Autodesk Inventor part; units mm, degrees
ref_plane "YZ Plane" through (0, 0, 0) normal (1, 0, 0) x (0, 1, 0)
ref_plane "XZ Plane" through (0, 0, 0) normal (0, 1, 0) x (-1, 0, 0)
ref_plane "XY Plane" through (0, 0, 0) normal (0, 0, 1) x (1, 0, 0)
sketch "Szkic1" plane through (0, 0, 0) normal (0, 0, 1) x (1, 0, 0)
  line L0 (11.5, -11.5) -> (-11.5, -11.5)
  line L1 (-11.5, -11.5) -> (-11.5, 11.5)
  line L2 (-11.5, 11.5) -> (11.5, 11.5)
  line L3 (11.5, 11.5) -> (11.5, -11.5)
  line L4 (11.5, -11.5) -> (-11.5, 11.5) construction
  line L5 (-11.5, -11.5) -> (11.5, 11.5) construction
  point P0 (0, 0)
  dimension "d0" = 23
  dimension "d1" = 23
extrude "Wyciągnięcie proste1" add sketch "Szkic1" along normal blind 23
fillet "Zaokrąglenie1" radius 0.5 12 edges at (0, 11.5, 23) (11.5, 11.5, 11.5) (11.5, 0, 23) (11.5, 0, 0) (11.5, -11.5, 11.5) (0, -11.5, 23) (0, -11.5, 0) (-11.5, -11.5, 11.5) (0, 11.5, 0) (-11.5, 11.5, 11.5) (-11.5, 0, 0) (-11.5, 0, 23)
sketch "Szkic2" plane through (0, 0, 23) normal (0, 0, 1) x (1, 0, 0)
  circle A0 centre (0, 0) radius 1.75
  circle A1 centre (0, 0) radius 2.25
  dimension "d5" = 3.5
  dimension "d6" = 4.5
extrude "Wyciągnięcie proste2" add sketch "Szkic2" along normal blind 1
fillet "Zaokrąglenie2" radius 1 1 edges at (-2.25, 0, 23)
properties part number "Kamera"
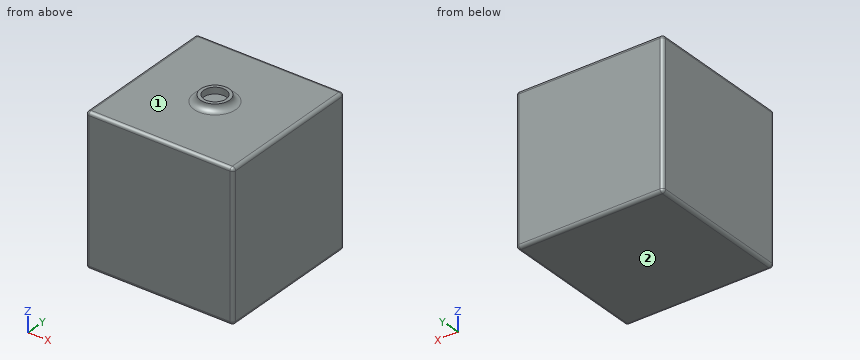
Work out the finished part from the listing and answer in its coordinate system (mm). Face numbers are marked on the shaded views. A direction names the side the tool comes from. Give positions to 0.01 mm unless a question says otherwise; leave off trailing zeros. Order: outer loops, then holes, each group sorted by start corner. A loop starts at its lowest first (then second) coordinate and runs counter-clockwise, first axis right, second up. Notation, with made-up numbers: M 1.25,49.25 L 24.25,49.25 A6 ccw 24.25,58.25 Z; hole C -9,-29.5 d2. An arc over 180 degrees is marked long. Return JSON: item names as keys, results as strings.
1) A tool of negligible diameter and unlimited length cuts with its end or side. For the marked faces 1 and 2, from which of +Z, -Z, +X, -X, +Y, -Y can it reach the whole face along a straight path? Write none if from no direction.
Resolved:
{"face 1": "+Z", "face 2": "-Z, +X, -X, +Y, -Y"}
2) Section A-A, the plane x = 4.75 is taken. Write down the section's boundary in (y, z), plus the area to 3 significant figures.
Resolved:
{"outline": "M -11.5,0.5 A0.5 ccw -11,0 L 11,0 A0.5 ccw 11.5,0.5 L 11.5,22.5 A0.5 ccw 11,23 L -11,23 A0.5 ccw -11.5,22.5 Z", "area": "529 mm^2"}
3) Straight lines are drawn through the part: line 1 along Z through (x, y) = (1.25, 1); line 2 along Y through (x, z) = (0, 23.7); line 3 along Y through (x, z) = (0, 23.3). For each, find the intervals that lie inside material, in ascending order. Write a range as [from, to].
Resolved:
{"line 1": "[0, 23]", "line 2": "[-2.3, -1.75], [1.75, 2.3]", "line 3": "[-2.54, -1.75], [1.75, 2.54]"}
4) Each of these flat-tipped pins is pushed along its axis until it touches: pin 1 (5 mm diameter, centred on x = 6.5, y = 1.5, fed in from -Z); pin 2 (1 mm diameter, centred on x = 0, y = 0.5, fed in from +Z); pin 3 (6.5 mm diameter, centred on x = -4, y = 4.5, fed in from +Z). Where does it stop, or does it pass through?
Resolved:
{"pin 1": "z = 0", "pin 2": "z = 23", "pin 3": "z = 23.12"}
